```python
from build123d import *

# Parameters (mm, degrees)
SKETCH2_W           = 44.25
SKETCH2_H           = 25
SKETCH2_W_2         = 30.25
SKETCH2_H_2         = 11.75
BOSS_EXTRUDE1_DEPTH = 1.5
SKETCH3_W           = 25
SKETCH3_H           = 2
BOSS_EXTRUDE2_DEPTH = 110
BOSS_EXTRUDE3_DEPTH = 25
BOSS_EXTRUDE4_DEPTH = 7.3
SKETCH6_W           = 1.5
SKETCH6_H           = 7.3
BOSS_EXTRUDE5_DEPTH = 112
SKETCH8_W           = 1.5
SKETCH8_H           = 5.3
BOSS_EXTRUDE6_DEPTH = 22
SKETCH9_W           = 6.2
SKETCH9_H           = 6.2
CUT_EXTRUDE1_DEPTH  = 2
SKETCH10_W          = 25
SKETCH10_H          = 110
CUT_EXTRUDE2_DEPTH  = 0.5
SKETCH11_W          = 25
SKETCH11_H          = 154.25
SKETCH11_W_2        = 22
SKETCH11_H_2        = 151.25
BOSS_EXTRUDE7_DEPTH = 13.2
SKETCH12_W          = 5.1
SKETCH12_H          = 1.2
CUT_EXTRUDE3_DEPTH  = 158.803873527
SKETCH13_W          = 5.1
SKETCH13_H          = 1.2
CUT_EXTRUDE4_DEPTH  = 158.803873527


with BuildPart() as part:
    # Sketch2 → Boss-Extrude1 (new body)
    with BuildSketch(Plane(origin=(0, 0, 0), x_dir=(0, 1, 0), z_dir=(0, 0, 1))):
        with Locations((22.125, 12.5)):
            Rectangle(SKETCH2_W, SKETCH2_H)
        with Locations((20.625, 12.5)):
            Rectangle(SKETCH2_W_2, SKETCH2_H_2, mode=Mode.SUBTRACT)
    extrude(amount=BOSS_EXTRUDE1_DEPTH)



with BuildPart() as body_2:
    # Sketch3 → Boss-Extrude2 (new body)
    with BuildSketch(Plane(origin=(0, 44.25, 0), x_dir=(-1, 0, 0), z_dir=(0, 1, 0))):
        with Locations((12.5, 2.5)):
            Rectangle(SKETCH3_W, SKETCH3_H)
    extrude(amount=BOSS_EXTRUDE2_DEPTH)


with BuildPart() as part_1:
    add(part.part)

    add(body_2.part)  # Boss-Extrude3 merges body 2
    # Sketch4 → Boss-Extrude3 (add)
    with BuildSketch(Plane.YZ):
        Polygon((44.25, 3.5), (44.25, 1.5), (42.25, 1.5), align=None)
    extrude(amount=-BOSS_EXTRUDE3_DEPTH)

    # Sketch5 → Boss-Extrude4 (add)
    with BuildSketch(Plane.XY.offset(1.5)):
        Polygon((-1.5, 42.25), (-1.5, 1.5), (-23.5, 1.5), (-23.5, 42.25), (-25, 42.25), (-25, 0), (0, 0), (0, 42.25), align=None)
    extrude(amount=BOSS_EXTRUDE4_DEPTH)

    # Sketch6 → Boss-Extrude5 (add)
    with BuildSketch(Plane(origin=(0, 42.25, 0), x_dir=(-1, 0, 0), z_dir=(0, 1, 0))):
        with Locations((24.25, 5.15)):
            Rectangle(SKETCH6_W, SKETCH6_H)
        with Locations((0.75, 5.15)):
            Rectangle(SKETCH6_W, SKETCH6_H)
    extrude(amount=BOSS_EXTRUDE5_DEPTH)

    # Sketch8 → Boss-Extrude6 (add)
    with BuildSketch(Plane.YZ.offset(-23.5)):
        with Locations((153.5, 6.15)):
            Rectangle(SKETCH8_W, SKETCH8_H)
    extrude(amount=BOSS_EXTRUDE6_DEPTH)

    # Sketch9 → Cut-Extrude1 (cut)
    with BuildSketch(Plane(origin=(0, 0, 1.5), x_dir=(1, 0, 0), z_dir=(0, 0, -1))):
        with Locations((-12.5, -141.75)):
            Rectangle(SKETCH9_W, SKETCH9_H)
        with Locations((-12.5, -114.25)):
            Rectangle(SKETCH9_W, SKETCH9_H)
        with Locations((-12.5, -56.75)):
            Rectangle(SKETCH9_W, SKETCH9_H)
        with Locations((-12.5, -84.25)):
            Rectangle(SKETCH9_W, SKETCH9_H)
    extrude(amount=-CUT_EXTRUDE1_DEPTH, mode=Mode.SUBTRACT)

    # Sketch10 → Cut-Extrude2 (cut)
    with BuildSketch(Plane(origin=(0, 0, 1.5), x_dir=(1, 0, 0), z_dir=(0, 0, -1))):
        with Locations((-12.5, -99.25)):
            Rectangle(SKETCH10_W, SKETCH10_H)
    extrude(amount=-CUT_EXTRUDE2_DEPTH, mode=Mode.SUBTRACT)

    # Sketch11 → Boss-Extrude7 (add)
    with BuildSketch(Plane.XY.offset(8.8)):
        with Locations((-12.5, 77.125)):
            Rectangle(SKETCH11_W, SKETCH11_H)
        with Locations((-12.5, 77.125)):
            Rectangle(SKETCH11_W_2, SKETCH11_H_2, mode=Mode.SUBTRACT)
    extrude(amount=BOSS_EXTRUDE7_DEPTH)

    # Sketch12 → Cut-Extrude3 (cut, through all)
    with BuildSketch(Plane.XZ):
        with Locations((-12.5, 17.5)):
            Rectangle(SKETCH12_W, SKETCH12_H)
    extrude(amount=-CUT_EXTRUDE3_DEPTH, mode=Mode.SUBTRACT)

    # Sketch13 → Cut-Extrude4 (cut, through all)
    with BuildSketch(Plane.YZ):
        with Locations((38.5625, 17.5)):
            Rectangle(SKETCH13_W, SKETCH13_H)
    cut_extrude4 = extrude(amount=-CUT_EXTRUDE4_DEPTH, mode=Mode.SUBTRACT)

    # Mirror1: Cut-Extrude4 across plane
    add(cut_extrude4.mirror(Plane(origin=(0, 77.125, 0), x_dir=(0, 0, 1), z_dir=(0, -1, 0))), mode=Mode.SUBTRACT)


solid = part_1.part
```
Work out the finished part from the listing and answer in its coordinate system (mm). A direction names the side the tool comes from. Give positions to 0.01 mm unless a question says otherwise; leave off trailing zeros. Write each loop counter-clockwise with the first axis right and the second up, starting at its lowest first coordinate (ties: lowest second). Pieces come first, ordered by that corner, then holes. Notation, with made-up numbers: (24, -10) -> (70, -10) arc R28 ccw to (70, 27) -> close; hole circle Ø9 at (55.25, -7.75). An arc over 180 degrees is marked (long way). Write item = value, one per line.
Q1. Consider line 1 along X through (y, z) = (60.5, 18.25); line 2 along Y through (x, z) = (-20.25, 12.75); line 3 along Z through (x, y) = (-12.5, 124). Determine where each line is inside the solid, lowest interval first.
Computed values:
line_1 = -25 to -23.5, -1.5 to 0
line_2 = 0 to 1.5, 152.75 to 154.25
line_3 = 2 to 3.5
Q2. For a pull along Y with two mould halves and no side action, classify faces 4 (the flat face through (-1.5, 76, 12)), 5 (the flat face through (-25, 76, 11)), 6 (the flat face through (-13, 154.25, 12)) as pulls with the +Y half, pulls with the -Y half, needs draft (parallel to the pull), parting line crosses it, or undercut.
Computed values:
face_4 = undercut
face_5 = needs draft
face_6 = pulls with the +Y half
Q3. A tool of negligible diameter and unlimited length cuts with its end or side. For faces 1 (the flat face through (-13, 98, 2)), 2 (the flat face through (-24, 77, 22)), 3 (the flat face through (-13, 1.5, 12)), from which of +Z, -Z, +X, -X, +Y, -Y can it reach the whole face along a straight path? Write none if from no direction.
Computed values:
face_1 = -Z, +X, -X, +Y
face_2 = +Z, +X, -X, +Y, -Y
face_3 = +Z
Q4. Section B-B on z = 10.5 is taken. Determine the outline of the cut face in (x, y), and give its area (3 significant figures).
Computed values:
outline = (-25, 0) -> (0, 0) -> (0, 154.25) -> (-25, 154.25) -> close; hole (-23.5, 1.5) -> (-1.5, 1.5) -> (-1.5, 152.75) -> (-23.5, 152.75) -> close
area = 529 mm^2
Q5. Flat-ended cylindrical pins translate along their axes: pin 1 Ø0.8 at (x, z) = (-13, 0.5) entering from +Y; pin 2 Ø5 at (x, y) = (-10, 84.5) entering from -Z. Find the tip coordinate at first contact, or state that the pin passes through.
Computed values:
pin_1 = 44.25
pin_2 = 2
Q6. Section A-A on y = 13 is taken. Determine the outline of the cut face in (x, z) (3 decimals), and give its area (3 significant figures).
Computed values:
outline = (-25, 0) -> (-18.375, 0) -> (-18.375, 1.5) -> (-23.5, 1.5) -> (-23.5, 22) -> (-25, 22) -> close; (-6.625, 0) -> (0, 0) -> (0, 22) -> (-1.5, 22) -> (-1.5, 1.5) -> (-6.625, 1.5) -> close
area = 81.4 mm^2
Q7. Section D-D on y = 70.5 is taken. Determine the outline of the cut face in (x, z).
Computed values:
outline = (-25, 2) -> (0, 2) -> (0, 22) -> (-1.5, 22) -> (-1.5, 3.5) -> (-23.5, 3.5) -> (-23.5, 22) -> (-25, 22) -> close
Q8. Section C-C on x = -5.25 is taken. Determine the outline of the cut face in (y, z).
Computed values:
outline = (0, 0) -> (44.25, 0) -> (44.25, 2) -> (154.25, 2) -> (154.25, 22) -> (152.75, 22) -> (152.75, 3.5) -> (44.25, 3.5) -> (42.25, 1.5) -> (1.5, 1.5) -> (1.5, 22) -> (0, 22) -> close
